Can you work these out from the model? Positions are in its coordinate system, mm. A direction names the side the tool comes from. Give positions to 0.01 mm unless a question says otherwise; leave off trailing zeros. Loops run counter-clockwise (first coordinate to the right, second up) from the corner with the lowest first, then second, coordinate; pieces in that order, holes last. Notation, with made-up numbers: M -6.5,22.5 L 1.5,22.5 A29 cw 1.5,52.5 Z; hole C 35,-12.75 d4. An arc over 180 degrees is marked long. Use CSV: the item, a comma, the result in double quotes.
from build123d import *

# Parameters (mm, degrees)
HOLE_WIZARD_M3_1_D       = 2.5
PATTERN_CIRCULAR_1_COUNT = 4


with BuildPart() as part:
    # Model → 旋转1 (revolve)
    with BuildSketch(Plane.XY, mode=Mode.PRIVATE) as revolve_1_sk:
        Polygon((-1.786351506, 28.377960803), (-1.786351506, -5.622039197), (0.713648494, -5.622039197), (0.713648494, 0.377960803), (1.213648494, 0.377960803), (1.213648494, 5.977960803), (2.213648494, 5.977960803), (2.213648494, 7.977960803), (8.213648494, 7.977960803), (8.213648494, 16.777960803), (2.213648494, 16.777960803), (2.213648494, 18.777960803), (1.213648494, 18.777960803), (1.213648494, 24.377960803), (0.713648494, 24.377960803), (0.713648494, 28.377960803), align=None)
    revolve(revolve_1_sk.sketch.rotate(Axis((-1.786351506, 28.377960803, 0), (0, -1, 0)), 90), axis=Axis((-1.786351506, 28.377960803, 0), (0, -1, 0)))

    # M3 螺纹孔1 (through all)
    with Locations(Plane(origin=(-1.786351506, 7.977960803, 7), x_dir=(0, 0, -1), z_dir=(0, -1, 0))):
        with Locations((0, 0)):
            hole_wizard_m3_1 = Hole(HOLE_WIZARD_M3_1_D / 2)

    # 阵列(圆周)1: M3 螺纹孔1 ×4 about axis
    pattern_circular_1_axis = Axis((-1.786351506, 0, 0), (0, 1, 0))
    for i in range(1, PATTERN_CIRCULAR_1_COUNT):
        add(hole_wizard_m3_1.rotate(pattern_circular_1_axis, i * 360 / PATTERN_CIRCULAR_1_COUNT), mode=Mode.SUBTRACT)


solid = part.part
Q1. I want a section at A-A, the plane x = -9. Please give me the cut outline in (y, z).
Model answer:
outline,"M 7.98,-6.93 L 16.78,-6.93 L 16.78,-1.23 L 7.98,-1.23 Z; M 7.98,1.23 L 16.78,1.23 L 16.78,6.93 L 7.98,6.93 Z"
Q2. I'm going to push flat-ended pins straight in: P1, Ø1.5, axis at y = 11, z = -5.5, coming from the -X side; P2, Ø10, axis at y = 7.5, z = -5.5, coming from the +X side; P3, Ø4, axis at x = 5.21, z = 0, coming from the -Y side; P4, Ø2, axis at x = -1.79, z = 7, coming from the -Y side. Where does each tip first touch, or does it pass through?
Model answer:
P1,"x = -10.59"
P2,"x = 8.2"
P3,"y = 7.98"
P4,"through"
Q3. I want a section at B-B, the plane z = 7. Please give me the cut outline in (x, y).
Model answer:
outline,"M -8.93,7.98 L -3.04,7.98 L -3.04,16.78 L -8.93,16.78 Z; M -0.54,7.98 L 5.36,7.98 L 5.36,16.78 L -0.54,16.78 Z"
Q4. For faces 5 (the cylindrical face through (1.142, 3.217, -0.65)), 6 (the cylindrical face through (-5.752, 17.792, -0.521)), 7 (the cylindrical face through (3.965, 12.44, -0.055)), which set-ups out of +Z, -Z, +X, -X, +Y, -Y let a thin tool reach every point of the face, with its end or its side?
Model answer:
face 5,"-Y"
face 6,"+Y"
face 7,"+Y, -Y"
Q5. I want a section at D-D, the plane z = 2. Please give me the cut outline in (x, y), then the cut area to 3 significant figures.
Model answer:
outline,"M -11.58,7.98 L -5.25,7.98 L -5.25,5.98 L -4.02,5.98 L -4.02,0.38 L -3.29,0.38 L -3.29,-5.62 L -0.29,-5.62 L -0.29,0.38 L 0.45,0.38 L 0.45,5.98 L 1.68,5.98 L 1.68,7.98 L 8.01,7.98 L 8.01,16.78 L 1.68,16.78 L 1.68,18.78 L 0.45,18.78 L 0.45,24.38 L -0.29,24.38 L -0.29,28.38 L -3.29,28.38 L -3.29,24.38 L -4.02,24.38 L -4.02,18.78 L -5.25,18.78 L -5.25,16.78 L -11.58,16.78 Z"
area,"280 mm2"
Q6. If we mould it in two halves opening along Z, with no side actions, what happens to faces 1 (the cylindrical face through (-1.84, 12.44, -5.75)), 2 (the cylindrical face through (1.142, 21.617, -0.65)), 3 (the flat face through (-1.9, 16.778, 4.3)), 4 (the cylindrical face through (-1.73, 12.44, 5.75))? For each: released by +Z, released by -Z, zero draft, split by the parting line, or undercut.
Model answer:
face 1,"undercut"
face 2,"split by the parting line"
face 3,"zero draft"
face 4,"undercut"
Q7. I want a section at C-C, the plane y = 9.5. Please give me the cut outline in (x, z).
Model answer:
outline,"C -1.79,0 d20; hole C -8.79,0 d2.5; hole C -1.79,-7 d2.5; hole C -1.79,7 d2.5; hole C 5.21,0 d2.5"
Q8. Please list where these lines run through material, in increasing order: L1, parallel to Y at x = -6.25, z = 4.5; L2, parallel to X at y = 13.5, z = 7; L3, parallel to Z at x = 5.5, y = 11. Write a range as from..to.
Model answer:
L1,"7.98..16.78"
L2,"-8.93..-3.04, -0.54..5.36"
L3,"-6.85..-1.22, 1.22..6.85"
